Verification items for the finished model (mm, model axes). Face numbers are marked on the shaded views. Round coordinates to 2 decimals unless told otherwise and drop trailing zeros. Write each loop counter-clockwise with the first axis right and the second up, starting at its lowest first coordinate (ties: lowest second). Pieces come first, ordered by that corner, then holes. Notation, with made-up numbers: M 58.25,15.5 L 73.25,15.5 A24 ccw 73.25,40.5 Z; hole C 4,9.25 d6. An arc over 180 degrees is marked long. Use a Markdown table: item, result. Add a question column.
from build123d import *

# Parameters (mm, degrees)
REVOLVE2_ANGLE    = 7
CIRPATTERN1_COUNT = 3


with BuildPart() as part:
    # Sketch1 → Revolve1 (revolve)
    with BuildSketch(Plane.XY, mode=Mode.PRIVATE) as revolve1_sk:
        Polygon((14, 0), (14.049784483, 2.75), (16.049784483, 2.75), (16, 0), align=None)
    revolve(revolve1_sk.sketch.rotate(Axis((0, 0, 0), (0, 1, 0)), 90), axis=Axis((0, 0, 0), (0, 1, 0)))  # turned: the seam where the file's is

    # Sketch2 → Revolve2 (revolve, symmetric)
    with BuildSketch(Plane.XY) as revolve2_sk:
        Polygon((14.049784483, 2.75), (16, 12), (18, 12), (16.049784483, 2.75), align=None)
    revolve2 = revolve(axis=Axis((0, 0, 0), (0, 1, 0)), revolution_arc=REVOLVE2_ANGLE / 2)
    revolve2 = revolve2 + revolve(revolve2_sk.sketch, axis=Axis((0, 0, 0), (0, -1, 0)), revolution_arc=REVOLVE2_ANGLE / 2)

    # CirPattern1: Revolve2 ×3 about axis
    cirpattern1_axis = Axis((0, 0, 0), (0, 1, 0))
    for i in range(1, CIRPATTERN1_COUNT):
        add(revolve2.rotate(cirpattern1_axis, i * 360 / CIRPATTERN1_COUNT))


solid = part.part
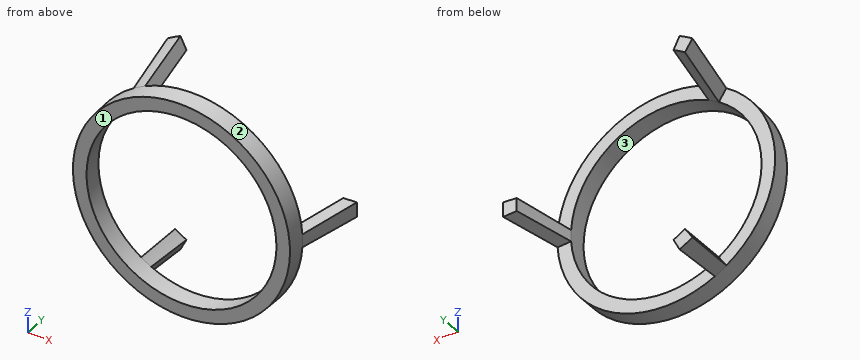
1. Scan lines: line 1 along X through (y, z) = (1.5, -2.5); line 2 along Y through (x, z) = (10, 11.5); line 3 along Z through (x, y) = (9.5, 1). Record each from-to range of solid material in increasing order. Write a range as from..to.
2. Release check for a two-part mould opening along Z. For the marked faces 1, 2 and 3 record: +Z half, -Z half, draft (parallel to the pull), parting line (faces both ways), or undercut.
3. Cross-section at A-A on y = 3.25. Enter the section's corners in (x, z).
4. Depth check by flat-ended pin: pin 1 Ø4 at (x, y) = (-11, 2) entering from +Z; pin 2 Ø16.5 at (x, z) = (6, 11.5) entering from +Y; pin 3 Ø3 at (x, y) = (13, 7.5) entering from -Z; pin 4 Ø6 at (y, z) = (3.5, 4.5) entering from -X. Enter the tip coordinate at first touch or a pass-through.
Answer:
| question | item | result |
|---|---|---|
| 1 | line 1 | x = -15.83..-13.8, 13.8..15.83 |
| 1 | line 2 | y = 0..2.75 |
| 1 | line 3 | z = -12.9..-10.31, 10.31..12.9 |
| 2 | face 1 | draft |
| 2 | face 2 | parting line |
| 2 | face 3 | undercut |
| 3 | outline | M -8.92,-13.47 A16.16 ccw -7.21,-14.46 L -6.32,-12.67 A14.16 cw -7.81,-11.8 Z; M -8.92,13.47 L -7.81,11.8 A14.16 cw -6.32,12.67 L -7.21,14.46 A16.16 ccw Z; M 14.13,-0.86 L 16.13,-0.99 A16.16 ccw 16.13,0.99 L 14.13,0.86 A14.16 cw Z |
| 4 | pin 1 | stops at z = 13.27 |
| 4 | pin 2 | stops at y = 2.75 |
| 4 | pin 3 | passes through |
| 4 | pin 4 | stops at x = -15.97 |
